Source: CAD feature listing. Evaluate the final solid. Frame: model axes, mm. A direction names the side the tool comes from. Round coordinates to 2 decimals unless told otherwise and drop trailing zeros. Order: outer loops, then holes, each group sorted by start corner. A loop starts at its lowest first (then second) coordinate and runs counter-clockwise, first axis right, second up. Notation, with made-up numbers: M -15.5,21.25 L 37.5,21.25 A29 ccw 37.5,54.25 Z; hole C 62.5,35.25 d2. An arc over 180 degrees is marked long. Use one line per item in the form item = value. Start each with the question number.
Q1. Material intervals for probe 1 along Z at (x, y) = (-56, 8); probe 2 along Z at (x, y) = (-48.5, 21); probe 3 along Z at (x, y) = (-8, 20.5), sorted ascending.
Q2. Contact query for flat-ended pins moving along their axis: pin 1 (4 mm diameter, centred on x = 35, z = 31, fed in from +Y); pin 2 (1 mm diameter, centred on x = 45, y = 5.5, fed in from +Z); pin 3 (1 mm diameter, centred on y = 23.5, z = 45.5, fed in from +X); pin 4 (1.7 mm diameter, centred on y = 12, z = -7.03, fed in from -X). Output: stop coordinate, or through.
Q3. Section C-C (x = 3.5). Return the cut outline in (y, z), plus the area to 3 significant figures.
Q4. Pull-direction query (X, two-part tool) for faces 4 (the cylindrical face through (34.427, 25.913, 48.655)), 5 (the flat face through (-50.326, 16, 2)), 6 (the flat face through (-13.914, 12, -26)); classes: pulls with the +X half, pulls with the -X half, needs draft (parallel to the pull), parting line crosses it, or undercut.
Q5. Section B-B (x = -57). Return the cut outline in (y, z).
Q6. Section A-A (x = 42.5). Return the cut outline in (y, z), plus the area to 3 significant figures.
Q7. Reachability of faces 1 (the flat face through (31.936, 12, 40)), 2 (the flat face through (39, 22.294, -20)), 3 (the flat face through (-9.573, 10, 31)) from +Z, -Z, +X, -X, +Y, -Y: full face, straight path, thin tool, end or side. Return the list, or none.
Q8. Section D-D (x = -32). Return the cut outline in (y, z), plus the area to 3 significant figures.
from build123d import *

# Parameters (mm, degrees)
SKETCH1_W            = 134
SKETCH1_H            = 55
BOSS_EXTRUDE1_DEPTH  = 5
BOSS_EXTRUDE2_DEPTH  = 14
SKETCH6_R            = 2
CUT_EXTRUDE2_DEPTH   = 16
BOSS_EXTRUDE4_DEPTH  = 10
SKETCH8_R            = 1.5
BOSS_EXTRUDE5_DEPTH  = 6
SKETCH9_W            = 9
SKETCH9_H            = 6
SKETCH9_R            = 0.666669423
CUT_EXTRUDE3_DEPTH   = 6
BOSS_EXTRUDE6_DEPTH  = 30
SKETCH11_W           = 26
SKETCH11_H           = 35
BOSS_EXTRUDE7_DEPTH  = 11
SKETCH12_R           = 2
CUT_EXTRUDE4_DEPTH   = 89.466034115
SKETCH13_W           = 29
SKETCH13_H           = 1
CUT_EXTRUDE5_DEPTH   = 23
BOSS_EXTRUDE8_DEPTH  = 12
SKETCH15_W           = 7.881166065
SKETCH15_H           = 6.31785274
BOSS_EXTRUDE9_DEPTH  = 8.206
SKETCH17_W           = 5
SKETCH17_H           = 42
BOSS_EXTRUDE10_DEPTH = 8.206
SKETCH18_W           = 27.737732315
SKETCH18_H           = 11
CUT_EXTRUDE6_DEPTH   = 5
SKETCH19_W           = 8.32170706
SKETCH19_H           = 17.542615134
SKETCH19_H_2         = 2.457384866
BOSS_EXTRUDE11_DEPTH = 25
SKETCH21_W           = 41.935962389
SKETCH21_H           = 5
BOSS_EXTRUDE12_DEPTH = 15
SKETCH22_R           = 2.7
CUT_EXTRUDE7_DEPTH   = 3.2
SKETCH23_R           = 1.5
CUT_EXTRUDE8_DEPTH   = 8.2
SKETCH24_R           = 2
CUT_EXTRUDE9_DEPTH   = 6.2
SKETCH25_R           = 2
CUT_EXTRUDE10_DEPTH  = 10.2
SKETCH26_W           = 4.703812025
SKETCH26_H           = 13.040944853
BOSS_EXTRUDE13_DEPTH = 25
SKETCH27_R           = 2
CUT_EXTRUDE11_DEPTH  = 11.2
SKETCH28_W           = 12.881166065
SKETCH28_H           = 42
BOSS_EXTRUDE14_DEPTH = 5
SKETCH29_R           = 1.5
CUT_EXTRUDE12_DEPTH  = 7
SKETCH30_R           = 2.75
CUT_EXTRUDE13_DEPTH  = 3
SKETCH31_W           = 15.85625148
SKETCH31_H           = 12.7
CUT_EXTRUDE14_DEPTH  = 8
FILLET1_R            = 10
FILLET2_R            = 10
FILLET3_R            = 10


with BuildPart() as part:
    # Sketch1 → Boss-Extrude1 (new body)
    with BuildSketch(Plane(origin=(0, 0, 0), x_dir=(1, 0, 0), z_dir=(0, 1, 0))):
        with Locations((-6.326180258, -10.214288954)):
            Rectangle(SKETCH1_W, SKETCH1_H)
    extrude(amount=BOSS_EXTRUDE1_DEPTH)

    # Sketch2 → Boss-Extrude2 (add)
    with BuildSketch(Plane(origin=(0, 5, 0), x_dir=(1, 0, 0), z_dir=(0, 1, 0))):
        Polygon((-73.326180258, 14.82832618), (-73.326180258, 11.82832618), (-50.326180258, 11.82832618), (-50.326180258, -17.17167382), (-73.326180258, -17.17167382), (-73.326180258, -20.17167382), (-47.326180258, -20.17167382), (-47.326180258, 14.82832618), align=None)
    extrude(amount=BOSS_EXTRUDE2_DEPTH)

    # Sketch6 → Cut-Extrude2 (cut)
    with BuildSketch(Plane(origin=(0, 5, 0), x_dir=(1, 0, 0), z_dir=(0, 1, 0))):
        with Locations(Location((-5.143804301, 11.824371315, 0), (0, 0, 270))):
            Circle(SKETCH6_R)
    extrude(amount=-CUT_EXTRUDE2_DEPTH, mode=Mode.SUBTRACT)

    # Sketch7 → Boss-Extrude4 (add)
    with BuildSketch(Plane(origin=(0, 5, 0), x_dir=(1, 0, 0), z_dir=(0, 1, 0))):
        Polygon((-9.572595602, -29.175628685), (12.857306, -29.175628685), (50.427404398, -29.175628685), (50.427404398, -33.25833673), (-9.572595602, -33.25833673), align=None)
    extrude(amount=BOSS_EXTRUDE4_DEPTH)

    # Sketch8 → Boss-Extrude5 (add)
    with BuildSketch(Plane(origin=(0, 5, 0), x_dir=(1, 0, 0), z_dir=(0, 1, 0))):
        with Locations(Location((46.72611237, 11.824371315, 0), (0, 0, 270))):
            Circle(SKETCH8_R)
    extrude(amount=BOSS_EXTRUDE5_DEPTH)

    # Sketch9 → Cut-Extrude3 (cut)
    with BuildSketch(Plane.ZY.offset(50.326180258)):
        with Locations((2.67167382, 12)):
            Rectangle(SKETCH9_W, SKETCH9_H)
        with Locations((-7.02832618, 12)):
            Circle(SKETCH9_R)
        with Locations((12.37167382, 12)):
            Circle(SKETCH9_R)
    extrude(amount=-CUT_EXTRUDE3_DEPTH, mode=Mode.SUBTRACT)

    # Sketch10 → Boss-Extrude6 (add)
    with BuildSketch(Plane(origin=(0, 0, 0), x_dir=(1, 0, 0), z_dir=(0, 1, 0))):
        Polygon((-73.326180258, 17.285711046), (-73.326180258, 22.285711046), (66.673819742, 22.285711046), (66.673819742, -42.714288954), (-73.326180258, -42.714288954), (-73.326180258, -37.714288954), (60.673819742, -37.714288954), (60.673819742, 17.285711046), align=None)
    extrude(amount=BOSS_EXTRUDE6_DEPTH)

    # Sketch11 → Boss-Extrude7 (add)
    with BuildSketch(Plane(origin=(0, 19, 0), x_dir=(1, 0, 0), z_dir=(0, 1, 0))):
        with Locations((-60.326180258, -2.67167382)):
            Rectangle(SKETCH11_W, SKETCH11_H)
    extrude(amount=BOSS_EXTRUDE7_DEPTH)

    # Sketch12 → Cut-Extrude4 (cut, through all)
    with BuildSketch(Plane(origin=(0, 5, 0), x_dir=(1, 0, 0), z_dir=(0, 1, 0))):
        with Locations(Location((-40.868568225, -32.116513497, 0), (0, 0, 270))):
            Circle(SKETCH12_R)
        with Locations(Location((-23.868568225, -32.116530453, 0), (0, 0, 270))):
            Circle(SKETCH12_R)
    extrude(amount=-CUT_EXTRUDE4_DEPTH, mode=Mode.SUBTRACT)

    # Sketch13 → Cut-Extrude5 (cut)
    with BuildSketch(Plane.ZY.offset(73.326180258)):
        with Locations((2.67167382, 19.5)):
            Rectangle(SKETCH13_W, SKETCH13_H)
    extrude(amount=-CUT_EXTRUDE5_DEPTH, mode=Mode.SUBTRACT)

    # Sketch14 → Boss-Extrude8 (add)
    with BuildSketch(Plane.XZ):
        Polygon((-13.914425371, -22.285711046), (46.65185498, -22.285711046), (46.65185498, -17.285711046), (-13.914425371, -17.285711046), (-18.914425371, -17.285711046), (-18.914425371, -22.285711046), align=None)
    extrude(amount=BOSS_EXTRUDE8_DEPTH)

    # Sketch15 → Boss-Extrude9 (add)
    with BuildSketch(Plane(origin=(0, 0, -22.285711046), x_dir=(-1, 0, 0), z_dir=(0, 0, -1))):
        with Locations((9.973842339, -8.84107363)):
            Rectangle(SKETCH15_W, SKETCH15_H)
    extrude(amount=BOSS_EXTRUDE9_DEPTH)

    # Sketch17 → Boss-Extrude10 (add)
    with BuildSketch(Plane(origin=(0, 0, -22.285711046), x_dir=(-1, 0, 0), z_dir=(0, 0, -1))):
        with Locations((16.414425371, 9)):
            Rectangle(SKETCH17_W, SKETCH17_H)
    extrude(amount=BOSS_EXTRUDE10_DEPTH)

    # Sketch18 → Cut-Extrude6 (cut)
    with BuildSketch(Plane.XY.offset(42.714288954)):
        with Locations((45.804953585, 12.5)):
            Rectangle(SKETCH18_W, SKETCH18_H)
    extrude(amount=-CUT_EXTRUDE6_DEPTH, mode=Mode.SUBTRACT)

    # Sketch19 → Boss-Extrude11 (add)
    with BuildSketch(Plane(origin=(0, 5, 0), x_dir=(1, 0, 0), z_dir=(0, 1, 0))):
        with Locations((-69.165326728, -28.942981387)):
            Rectangle(SKETCH19_W, SKETCH19_H)
        with Locations((-69.165326728, 16.057018613)):
            Rectangle(SKETCH19_W, SKETCH19_H_2)
    extrude(amount=BOSS_EXTRUDE11_DEPTH)

    # Sketch21 → Boss-Extrude12 (add)
    with BuildSketch(Plane.XY.offset(42.714288954)):
        with Locations((45.705838548, 27.5)):
            Rectangle(SKETCH21_W, SKETCH21_H)
    extrude(amount=BOSS_EXTRUDE12_DEPTH)

    # Sketch22 → Cut-Extrude7 (cut)
    with BuildSketch(Plane(origin=(0, 30, 0), x_dir=(1, 0, 0), z_dir=(0, 1, 0))):
        with Locations(Location((32.939337155, -48.85061207, 0), (0, 0, 270))):
            Circle(SKETCH22_R)
        with Locations(Location((60.22852181, -48.85061207, 0), (0, 0, 270))):
            Circle(SKETCH22_R)
    extrude(amount=-CUT_EXTRUDE7_DEPTH, mode=Mode.SUBTRACT)

    # Sketch23 → Cut-Extrude8 (cut)
    with BuildSketch(Plane(origin=(0, 30, 0), x_dir=(1, 0, 0), z_dir=(0, 1, 0))):
        with Locations(Location((60.22852181, -48.85061207, 0), (0, 0, 270))):
            Circle(SKETCH23_R)
        with Locations(Location((32.939337155, -48.85061207, 0), (0, 0, 270))):
            Circle(SKETCH23_R)
    extrude(amount=-CUT_EXTRUDE8_DEPTH, mode=Mode.SUBTRACT)

    # Sketch24 → Cut-Extrude9 (cut)
    with BuildSketch(Plane.XY.offset(42.714288954)):
        with Locations((-69.643270331, 26.922023127)):
            Circle(SKETCH24_R)
    extrude(amount=-CUT_EXTRUDE9_DEPTH, mode=Mode.SUBTRACT)

    # Sketch25 → Cut-Extrude10 (cut)
    with BuildSketch(Plane(origin=(0, 30, 0), x_dir=(1, 0, 0), z_dir=(0, 1, 0))):
        with Locations(Location((-68.301285916, -29.073958674, 0), (0, 0, 270))):
            Circle(SKETCH25_R)
    extrude(amount=-CUT_EXTRUDE10_DEPTH, mode=Mode.SUBTRACT)

    # Sketch26 → Boss-Extrude13 (add)
    with BuildSketch(Plane(origin=(0, 5, 0), x_dir=(1, 0, 0), z_dir=(0, 1, 0))):
        with Locations((58.32191373, 10.765238619)):
            Rectangle(SKETCH26_W, SKETCH26_H)
    extrude(amount=BOSS_EXTRUDE13_DEPTH)

    # Sketch27 → Cut-Extrude11 (cut)
    with BuildSketch(Plane(origin=(0, 30, 0), x_dir=(1, 0, 0), z_dir=(0, 1, 0))):
        with Locations(Location((61.565901952, 12.965958555, 0), (0, 0, 270))):
            Circle(SKETCH27_R)
    extrude(amount=-CUT_EXTRUDE11_DEPTH, mode=Mode.SUBTRACT)

    # Sketch28 → Boss-Extrude14 (add)
    with BuildSketch(Plane(origin=(0, 0, -30.491711046), x_dir=(-1, 0, 0), z_dir=(0, 0, -1))):
        with Locations((12.473842339, 9)):
            Rectangle(SKETCH28_W, SKETCH28_H)
    extrude(amount=BOSS_EXTRUDE14_DEPTH)

    # Sketch29 → Cut-Extrude12 (cut)
    with BuildSketch(Plane(origin=(0, -5.68214726, 0), x_dir=(1, 0, 0), z_dir=(0, 1, 0))):
        with Locations(Location((-9.973842338, 26.388711046, 0), (0, 0, 270))):
            Circle(SKETCH29_R)
    extrude(amount=-CUT_EXTRUDE12_DEPTH, mode=Mode.SUBTRACT)

    # Sketch30 → Cut-Extrude13 (cut)
    with BuildSketch(Plane.XZ.offset(12)):
        with Locations(Location((-9.973842338, -26.388711046, 0), (0, 0, 270))):
            Circle(SKETCH30_R)
    extrude(amount=-CUT_EXTRUDE13_DEPTH, mode=Mode.SUBTRACT)

    # Sketch31 → Cut-Extrude14 (cut)
    with BuildSketch(Plane(origin=(0, 0, -22.285711046), x_dir=(-1, 0, 0), z_dir=(0, 0, -1))):
        with Locations((-38.72372924, 15.943526368)):
            Rectangle(SKETCH31_W, SKETCH31_H)
    extrude(amount=-CUT_EXTRUDE14_DEPTH, mode=Mode.SUBTRACT)

    # Fillet1
    # the kernel refuses this fillet: 10 mm, written as the material it adds along each edge
    with BuildSketch(Plane(origin=(46.65185498, 0, -17.285711046), x_dir=(0, 0, 1), z_dir=(-1, 0, 0))) as fillet1_piece_1_section:
        with BuildLine():
            CenterArc((FILLET1_R, -FILLET1_R), FILLET1_R, 90, 90)
            Line((0, -FILLET1_R), (0, 0))
            Line((0, 0), (FILLET1_R, 0))
        make_face()
    fillet1_piece_1 = extrude(amount=65.56628035, mode=Mode.PRIVATE)
    fillet1_piece_1 = fillet1_piece_1 - Plane(origin=(-5.143804301, -2.281344891, -11.824371315), x_dir=(0, 0, 1), z_dir=(0, 1, 0)) * Cylinder(2, 172, mode=Mode.PRIVATE)
    add(fillet1_piece_1)

    # Fillet2
    fillet2_edges = [part.edges().sort_by_distance(p)[0] for p in [
        (-18.914425371, 0, -14.785711046),
    ]]
    fillet(fillet2_edges, radius=FILLET2_R)

    # Fillet3
    fillet3_edges = [part.edges().sort_by_distance(p)[0] for p in [
        (46.65185498, 0, -14.785711046),
    ]]
    fillet(fillet3_edges, radius=FILLET3_R)


solid = part.part
Results list:
q1.probe_1 = -22.29 to -17.29, -14.83 to -11.83, 17.17 to 20.17, 37.71 to 42.71
q1.probe_2 = -22.29 to -17.29, -14.83 to 20.17, 37.71 to 42.71
q1.probe_3 = -35.49 to -30.49, -22.29 to -17.29, 37.71 to 42.71
q2.pin_1 = 15
q2.pin_2 = 42.71
q2.pin_3 = through
q2.pin_4 = -50.33
q3.outline = M -12,-22.29 L 30,-22.29 L 30,-17.29 L 5,-17.29 L 5,29.18 L 15,29.18 L 15,33.26 L 5,33.26 L 5,37.71 L 30,37.71 L 30,42.71 L 0,42.71 L 0,-7.29 A10 cw -10,-17.29 L -12,-17.29 Z
q3.area = 697 mm2
q4.face_4 = undercut
q4.face_5 = pulls with the -X half
q4.face_6 = pulls with the +X half
q5.outline = M 0,-22.29 L 30,-22.29 L 30,-17.29 L 5,-17.29 L 5,-14.83 L 30,-14.83 L 30,20.17 L 5,20.17 L 5,37.71 L 30,37.71 L 30,42.71 L 0,42.71 Z; hole M 5,-11.83 L 20,-11.83 L 20,17.17 L 5,17.17 Z
q6.outline = M -12,-22.29 L 9.59,-22.29 L 9.59,-17.29 L 5,-17.29 L 5,29.18 L 15,29.18 L 15,33.26 L 5,33.26 L 5,37.71 L 7,37.71 L 7,42.71 L 0,42.71 L 0,-7.29 A10 cw -10,-17.29 L -12,-17.29 Z; M 18,37.71 L 30,37.71 L 30,57.71 L 25,57.71 L 25,42.71 L 18,42.71 Z; M 22.29,-22.29 L 30,-22.29 L 30,-17.29 L 22.29,-17.29 Z
q6.area = 654 mm2
q7.face_1 = +Z
q7.face_2 = -Z
q7.face_3 = +Y
q8.outline = M 0,-22.29 L 30,-22.29 L 30,-17.29 L 5,-17.29 L 5,37.71 L 30,37.71 L 30,42.71 L 0,42.71 Z
q8.area = 575 mm2
